```python
from build123d import *

# Parameters (mm, degrees)
BOSS_EXTRUDE1_DEPTH      = 10
SKETCH2_W                = 20
SKETCH2_H                = 10
BOSS_EXTRUDE2_DEPTH      = 10
BOSS_EXTRUDE3_DEPTH      = 5
BOSS_EXTRUDE4_DEPTH      = 2
BOSS_EXTRUDE4_DEPTH_BACK = 2
FILLET1_R                = 1
SKETCH6_R                = 3.175
CUT_EXTRUDE1_DEPTH       = 90.841967072
SKETCH8_W                = 55.480567722
SKETCH8_H                = 48.561795017
CUT_EXTRUDE2_DEPTH       = 2.75


with BuildPart() as part:
    # Sketch1 → Boss-Extrude1 (new body)
    with BuildSketch(Plane(origin=(0, 0, 0), x_dir=(1, 0, 0), z_dir=(0, 1, 0))):
        with BuildLine():
            Line((-13.509053295, -10.59136074), (-14.375325888, -11.091503454))
            ThreePointArc((-14.375325888, -11.091503454), (-15.870504116, -11.297182897), (-17.083695431, -10.39939183))
            ThreePointArc((-17.083695431, -10.39939183), (-19.377302502, 4.951782281), (-10, 17.320508076))
            Line((-10, 17.320508076), (-10, 21.320508076))
            Line((-10, 21.320508076), (2.687202796, 21.320508076))
            Line((2.687202796, 21.320508076), (10, 21.320508076))
            Line((10, 21.320508076), (10, 17.320508076))
            ThreePointArc((10, 17.320508076), (18.538798966, 7.504194355), (19.232390566, -5.487727502))
            ThreePointArc((19.232390566, -5.487727502), (18.059570944, -6.792834648), (16.309151509, -6.671005559))
            Line((16.309151509, -6.671005559), (15.414666731, -6.154574532))
            ThreePointArc((15.414666731, -6.154574532), (14.566381317, -5.186618632), (14.483529469, -3.902226816))
            ThreePointArc((14.483529469, -3.902226816), (-2.130312968, 14.847954965), (-12.802105849, -7.817038176))
            ThreePointArc((-12.802105849, -7.817038176), (-12.570985303, -9.353164625), (-13.509053295, -10.59136074))
        make_face()
    extrude(amount=BOSS_EXTRUDE1_DEPTH)

    # Sketch2 → Boss-Extrude2 (add)
    with BuildSketch(Plane(origin=(0, 0, -21.320508076), x_dir=(-1, 0, 0), z_dir=(0, 0, -1))):
        with Locations((0, 5)):
            Rectangle(SKETCH2_W, SKETCH2_H)
    extrude(amount=BOSS_EXTRUDE2_DEPTH)

    # Sketch3 → Boss-Extrude3 (add)
    with BuildSketch(Plane(origin=(0, 0, -31.320508076), x_dir=(-1, 0, 0), z_dir=(0, 0, -1))):
        with BuildLine():
            Line((-15, 75), (15, 75))
            ThreePointArc((15, 75), (22.071067812, 72.071067812), (25, 65))
            Line((25, 65), (25, 10))
            ThreePointArc((25, 10), (22.071067812, 2.928932188), (15, 0))
            Line((15, 0), (-15, 0))
            ThreePointArc((-15, 0), (-22.071067812, 2.928932188), (-25, 10))
            Line((-25, 10), (-25, 65))
            ThreePointArc((-25, 65), (-22.071067812, 72.071067812), (-15, 75))
        make_face()
    extrude(amount=BOSS_EXTRUDE3_DEPTH)

    # Sketch4 → Boss-Extrude4 (add, two sides: drawn at the far end of the back side and taken through both)
    with BuildSketch(Plane.ZY.offset(-BOSS_EXTRUDE4_DEPTH_BACK)):
        Polygon((-22.311101636, 10), (-31.320508076, 35), (-31.320508076, 10), align=None)
    extrude(amount=BOSS_EXTRUDE4_DEPTH + BOSS_EXTRUDE4_DEPTH_BACK)

    # Fillet1
    fillet1_edges = [part.edges().sort_by_distance(p)[0] for p in [
        (2, 22.5, -26.815804856),
        (-2, 22.5, -26.815804856),
    ]]
    fillet(fillet1_edges, radius=FILLET1_R)

    # Sketch6 → Cut-Extrude1 (cut, through all)
    with BuildSketch(Plane.XY.offset(-31.320508076)):
        with Locations((-15, 65)):
            Circle(SKETCH6_R)
        with Locations((15, 65)):
            Circle(SKETCH6_R)
        with Locations((15, 20)):
            Circle(SKETCH6_R)
        with Locations((-15, 20)):
            Circle(SKETCH6_R)
    extrude(amount=-CUT_EXTRUDE1_DEPTH, mode=Mode.SUBTRACT)

    # Sketch8 → Cut-Extrude2 (cut)
    with BuildSketch(Plane.XZ):
        with Locations((-0.773192615, -7.039610568)):
            Rectangle(SKETCH8_W, SKETCH8_H)
    extrude(amount=-CUT_EXTRUDE2_DEPTH, mode=Mode.SUBTRACT)


solid = part.part
```
Verification items for the finished model (mm, model axes). A direction names the side the tool comes from. Coordinates: 2 decimals unless noted, no trailing zeros. Write each loop counter-clockwise with the first axis right and the second up, starting at its lowest first coordinate (ties: lowest second). Pieces come first, ordered by that corner, then holes. Notation, with made-up numbers: M 41.25,32.25 L 72.25,32.25 A18 ccw 72.25,40.25 Z; hole C 22,10 d6. An arc over 180 degrees is marked long. Answer as a JSON object with one key per item and string values. Group by question number.
(1) Cross-section at D-D, the plane y = 8.5. Record the cut outline in (x, z), and give its area (3 significant figures).
(2) Release check for a two-part mould opening along Z. For faces 4 (the face through (-19.43, 6.32, -4.74)), 5 (the face through (0, 10, -19)), 6 (the face through (-12.566, 6.324, 9.331)), 7 (the face through (0.014, 22.325, -26.753)) record: +Z half, -Z half, draft (parallel to the pull), parting line (faces both ways), or undercut.
(3) Cross-section at C-C, the plane y = 59.5. Record the cut outline in (x, z).
(4) Cross-section at B-B, the plane x = 0. Record the cut outline in (y, z).
(5) Material ranges on line 1 (Y direction, x = 15, z = -34) (3 decimals); line 2 (Z direction, x = -4, y = 51.5); line 3 (X direction, y = 5.75, z = 0), recorded low to high.
(6) Tool access check on faces 1 (the face through (-10, 6, -24)), 2 (the face through (17.93, 18.78, -33.79)), 3 (the face through (-2, 16, -29)). Record the directions out of +Z, -Z, +X, -X, +Y, -Y that give a thin tool (end or side, any length) a straight path to the whole face; none if there is none.
(7) Cross-section at A-A, the plane z = 0. Record the cut outline in (x, y), and give its area (3 significant figures).
(8) Gauge pin test, flat ends, axial feed: pin 1 (6 mm diameter, centred on y = 15.5, z = -20, fed in from +X); pin 2 (1 mm diameter, centred on x = -13.5, z = -12, fed in from +Y); pin 3 (2 mm diameter, centred on x = -18.5, y = 52.5, fed in from +Z); pin 4 (8.5 mm diameter, centred on y = 19.5, z = -26, fed in from +X). Record the tip position at first contact, or that the pin passes through.
Reply:
{
 "1": {"outline": "M -24.89,-36.32 L 24.89,-36.32 L 24.89,-31.32 L 10,-31.32 L 10,-17.32 A20 ccw 19.23,5.49 A2 ccw 16.31,6.67 L 15.41,6.15 A2 ccw 14.48,3.9 A15 cw long -12.8,7.82 A2 ccw -13.51,10.59 L -14.38,11.09 A2 ccw -17.08,10.4 A20 ccw -10,-17.32 L -10,-31.32 L -24.89,-31.32 Z", "area": "856 mm²"},
 "2": {"face 4": "undercut", "face 5": "draft", "face 6": "undercut", "face 7": "+Z half"},
 "3": {"outline": "M -25,-36.32 L 25,-36.32 L 25,-31.32 L -25,-31.32 Z"},
 "4": {"outline": "M 0,-36.32 L 75,-36.32 L 75,-31.32 L 35,-31.32 L 10,-22.31 L 10,-15 L 2.75,-15 L 2.75,-31.32 L 0,-31.32 Z"},
 "5": {"line 1": "0 to 16.825, 23.175 to 61.825, 68.175 to 75", "line 2": "-36.32 to -31.32", "line 3": "-20 to -15, 15 to 20"},
 "6": {"face 1": "-X, +Y, -Y", "face 2": "+Z, -Z", "face 3": "+Z, -X, +Y"},
 "7": {"outline": "M -20,2.75 L -15,2.75 L -15,10 L -20,10 Z; M 15,2.75 L 20,2.75 L 20,10 L 15,10 Z", "area": "72.5 mm²"},
 "8": {"pin 1": "through", "pin 2": "y = 10", "pin 3": "z = -31.32", "pin 4": "x = 2"}
}
